Could you check a few things on this drawing? It's one solid part, dimensions in mm from its lowest x, y, z. A direction names the side the tool comes from. Give positions to 0.01 mm unless a question says otherwise; leave off trailing zeros. Write each loop counter-clockwise with the first axis right and the second up, starting at its lowest first coordinate (ties: lowest second). Pieces come first, ordered by that corner, then holes. Notation, with made-up numbers: (33, -25.5) -> (55, -25.5) arc R19 ccw to (55, -6.5) -> close; hole circle Ø1 at (50, 51). An arc over 180 degrees is marked (long way). Answer as CSV lines item,"result". Start each with the question number.
1. If we section it at C-C on z = 4.5: Write out the boundary of the cut face in (x, y).
2. I'm going to push flat-ended pins straight in: P1, Ø3, axis at y = 8, z = 16, coming from the -X side; P2, Ø6.5, axis at x = 10.5, y = 10.5, coming from the -Z side; P3, Ø1.5, axis at x = 7, y = 8.5, coming from the -Z side; P4, Ø5, axis at x = 6.5, z = 19.5, coming from the +Y side. Where does each tip first touch, or does it pass through?
3. If we mould it in two halves opening along Y, with no side actions, what happens to the marked faces 1, 2 and 3? For each: pulls with the +Y half, pulls with the -Y half, needs draft (parallel to the pull), parting line crosses it, or undercut.
4. If we section it at A-A on y = 10: Write out the boundary of the cut face in (x, z), plus the area to 3 significant figures.
5. On a 3-axis mill with a long thin cutter (end or side, diameter ignored), from which of +Z, -Z, +X, -X, +Y, -Y can I reach the whole of each face in a straight line? I mean the marked faces 4 and 5. Say none if no direction works.
6. I need wall thicknesses on line 1 (Y direction, x = 10, z = 22); line 2 (Z direction, x = 9, y = 11.5); line 3 (Y direction, x = 10, z = 6.5). Which ranges of each line are inside material? Lowest first, please. Write a range as [from, to].
7. If we section it at D-D on z = 13.75: Write out the boundary of the cut face in (x, y), plus the area to 3 significant figures.
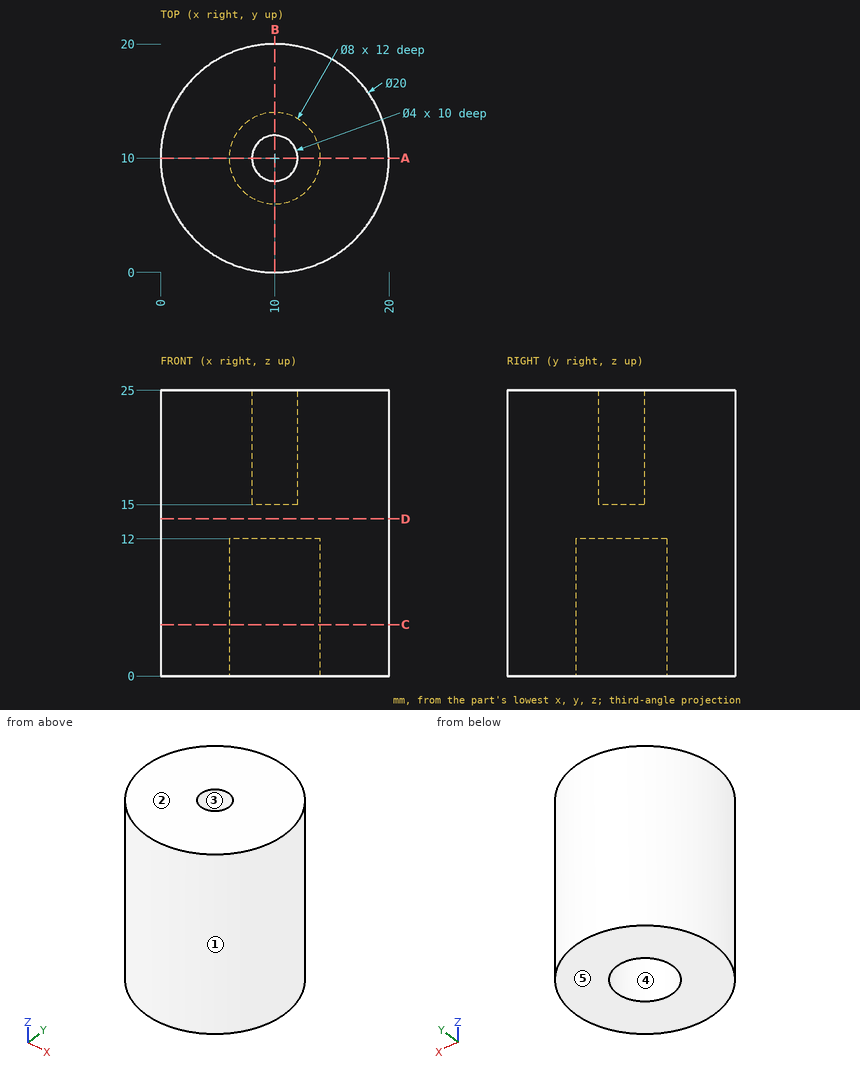
Computed values:
1,outline,"circle Ø20 at (10, 10); hole circle Ø8 at (10, 10)"
2,P1,"stops at x = 0.01"
2,P2,"stops at z = 12"
2,P3,"stops at z = 0"
2,P4,"stops at y = 19.95"
3,face 1,"parting line crosses it"
3,face 2,"needs draft"
3,face 3,"undercut"
4,outline,"(0, 0) -> (6, 0) -> (6, 12) -> (14, 12) -> (14, 0) -> (20, 0) -> (20, 25) -> (12, 25) -> (12, 15) -> (8, 15) -> (8, 25) -> (0, 25) -> close"
4,area,"364 mm2"
5,face 4,"-Z"
5,face 5,"-Z, +X, -X, +Y, -Y"
6,line 1,"y = [0, 8], [12, 20]"
6,line 2,"z = [12, 15]"
6,line 3,"y = [0, 6], [14, 20]"
7,outline,"circle Ø20 at (10, 10)"
7,area,"314 mm2"
